from build123d import *

# Parameters (mm, degrees)
SKETCH1_R           = 16.5
SKETCH1_R_2         = 7.5
BOSS_EXTRUDE1_DEPTH = 3.175
FILLET1_R           = 0.1
SKETCH2_R           = 1.89865
CUT_EXTRUDE1_DEPTH  = 24.549535558
CIRPATTERN1_COUNT   = 8


with BuildPart() as part:
    # Sketch1 → Boss-Extrude1 (new body)
    with BuildSketch(Plane(origin=(0, 0, 0), x_dir=(1, 0, 0), z_dir=(0, 1, 0))):
        with Locations(Location((0, 0, 0), (0, 0, 270))):
            Circle(SKETCH1_R)
        with Locations(Location((0, 0, 0), (0, 0, 270))):
            Circle(SKETCH1_R_2, mode=Mode.SUBTRACT)
    extrude(amount=BOSS_EXTRUDE1_DEPTH)

    # Fillet1
    fillet1_edges = [part.edges().sort_by_distance(p)[0] for p in [
        (0, 0, -7.5),
        (0, 3.175, -7.5),
    ]]
    fillet(fillet1_edges, radius=FILLET1_R)

    # Sketch2 → Cut-Extrude1 (cut, through all)
    with BuildSketch(Plane(origin=(0, 3.175, 0), x_dir=(-1, 0, 0), z_dir=(0, 1, 0))):
        with Locations(Location((0, -13.5, 0), (0, 0, 90))):
            Circle(SKETCH2_R)
    cut_extrude1 = extrude(amount=-CUT_EXTRUDE1_DEPTH, mode=Mode.SUBTRACT)

    # CirPattern1: Cut-Extrude1 ×8 about axis
    cirpattern1_axis = Axis((0, 0, 0), (0, 1, 0))
    for i in range(1, CIRPATTERN1_COUNT):
        add(cut_extrude1.rotate(cirpattern1_axis, i * 360 / CIRPATTERN1_COUNT), mode=Mode.SUBTRACT)


solid = part.part
Design review of the part built by this model. Coordinates are the model's own, in mm. Give positions to 0.01 mm unless a question says otherwise; leave off trailing zeros. Write each loop counter-clockwise with the first axis right and the second up, starting at its lowest first coordinate (ties: lowest second). Pieces come first, ordered by that corner, then holes. Notation, with made-up numbers: M -19.5,-6.5 L 31.5,-6.5 A7 ccw 31.5,5.5 Z; hole C -35.5,39 d7. An arc over 180 degrees is marked long. Return JSON: item names as keys, results as strings. Group by question number.
Item 1: The part is to be moulded in two halves that separate along X. For faces 1 (the flat face through (-7.1, 3.175, 3.4)), 2 (the cylindrical face through (0.33, 1.567, -7.493)), 3 (the cylindrical face through (-16.108, 1.565, -3.577)), say which applies: pulls with the +X half, pulls with the -X half, needs draft (parallel to the pull), parting line crosses it, or undercut.
Item 2: Take a section at C-C (z = -13.5). Give the boundary of the cut face in (x, y) (3 decimals).
Item 3: Take a section at D-D (x = 13.5). Give the boundary of the cut face in (y, z) (3 decimals), plus the area to 3 significant figures.
Item 4: Wall thickness on line 1 along Z through (x, y) = (1.5, 1.55); line 2 along X through (y, z) = (1.8, -0.5); line 3 along Z through (x, y) = (-15, 2.8): over which ranges is each line inside the solid? List them lowest first.
Item 5: Take a section at B-B (x = 0). Give the boundary of the cut face in (y, z) (3 decimals).
Item 6: Take a section at A-A (z = 0). Give the boundary of the cut face in (x, y) (3 decimals).
Return value:
{
 "1": {"face 1": "needs draft", "face 2": "undercut", "face 3": "parting line crosses it"},
 "2": {"outline": "M -9.487,0 L -1.899,0 L -1.899,3.175 L -9.487,3.175 Z; M 1.899,0 L 9.487,0 L 9.487,3.175 L 1.899,3.175 Z"},
 "3": {"outline": "M 0,-9.487 L 3.175,-9.487 L 3.175,-1.899 L 0,-1.899 Z; M 0,1.899 L 3.175,1.899 L 3.175,9.487 L 0,9.487 Z", "area": "48.2 mm2"},
 "4": {"line 1": "z = -16.43 to -14.66, -12.34 to -7.35, 7.35 to 12.34, 14.66 to 16.43", "line 2": "x = -16.49 to -15.33, -11.67 to -7.48, 7.48 to 11.67, 15.33 to 16.49", "line 3": "z = -6.87 to -1.16, 1.16 to 6.87"},
 "5": {"outline": "M 0,-16.5 L 3.175,-16.5 L 3.175,-15.399 L 0,-15.399 Z; M 0,-11.601 L 3.175,-11.601 L 3.175,-7.6 A0.1 ccw 3.075,-7.5 L 0.1,-7.5 A0.1 ccw 0,-7.6 Z; M 0,7.6 A0.1 ccw 0.1,7.5 L 3.075,7.5 A0.1 ccw 3.175,7.6 L 3.175,11.601 L 0,11.601 Z; M 0,15.399 L 3.175,15.399 L 3.175,16.5 L 0,16.5 Z"},
 "6": {"outline": "M -16.5,0 L -15.399,0 L -15.399,3.175 L -16.5,3.175 Z; M -11.601,0 L -7.6,0 A0.1 ccw -7.5,0.1 L -7.5,3.075 A0.1 ccw -7.6,3.175 L -11.601,3.175 Z; M 7.5,0.1 A0.1 ccw 7.6,0 L 11.601,0 L 11.601,3.175 L 7.6,3.175 A0.1 ccw 7.5,3.075 Z; M 15.399,0 L 16.5,0 L 16.5,3.175 L 15.399,3.175 Z"}
}
